Geometry check sheet. Reference: the model listing, model coordinates, mm. A direction names the side the tool comes from. Coordinates: 2 decimals unless noted, no trailing zeros. Write each loop counter-clockwise with the first axis right and the second up, starting at its lowest first coordinate (ties: lowest second). Pieces come first, ordered by that corner, then holes. Notation, with made-up numbers: M 43,-11 L 72,-11 A15 ccw 72,-2 Z; hole C -9.75,74 d11. An arc over 180 degrees is marked long. Write item = value, one per line. Start each with the question number.
```python
from build123d import *

# Parameters (mm, degrees)
BOSS_EXTRUDE1_DEPTH                        = 10
SKETCH3_R                                  = 4.5
CUT_EXTRUDE1_DEPTH                         = 44.28394626
MIRROR1_AT_THE_SECOND_PLANE_COPY_1_SKETC_R = 4.5
MIRROR1_AT_THE_SECOND_PLANE_COPY_1_DEPTH   = 44.28394626


with BuildPart() as part:
    # Sketch1 → Revolve1 (revolve)
    with BuildSketch(Plane.XY, mode=Mode.PRIVATE) as revolve1_sk:
        with BuildLine():
            Line((0, 9.5), (3.481747944, 9.5))
            ThreePointArc((3.481747944, 9.5), (3.98343056, 9.436056443), (4.453033806, 9.248314552))
            Line((4.453033806, 9.248314552), (7.6, 7.5))
            Line((7.6, 7.5), (7.6, -4.5))
            Line((7.6, -4.5), (17, -4.5))
            Line((17, -4.5), (17, -9.5))
            Line((17, -9.5), (7.6, -9.5))
            Line((7.6, -9.5), (0, -9.5))
            Line((0, -9.5), (0, 9.5))
        make_face()
    revolve(revolve1_sk.sketch.rotate(Axis((0, 9.5, 0), (0, -1, 0)), 90), axis=Axis((0, 9.5, 0), (0, -1, 0)))

    # Sketch2 → Boss-Extrude1 (add)
    with BuildSketch(Plane.XZ.offset(9.5)):
        with BuildLine():
            Line((17.5, 27.5), (-17.5, 27.5))
            ThreePointArc((-17.5, 27.5), (-24.571067812, 24.571067812), (-27.5, 17.5))
            Line((-27.5, 17.5), (-27.5, -17.5))
            ThreePointArc((-27.5, -17.5), (-24.571067812, -24.571067812), (-17.5, -27.5))
            Line((-17.5, -27.5), (17.5, -27.5))
            ThreePointArc((17.5, -27.5), (24.571067812, -24.571067812), (27.5, -17.5))
            Line((27.5, -17.5), (27.5, 17.5))
            ThreePointArc((27.5, 17.5), (24.571067812, 24.571067812), (17.5, 27.5))
        make_face()
    extrude(amount=BOSS_EXTRUDE1_DEPTH)

    # Sketch3 → Cut-Extrude1 (cut, through all)
    with BuildSketch(Plane(origin=(0, -9.5, 0), x_dir=(1, 0, 0), z_dir=(0, 1, 0))):
        with Locations(Location((-17.5, 17.5, 0), (0, 0, 270))):
            Circle(SKETCH3_R)
    cut_extrude1 = extrude(amount=-CUT_EXTRUDE1_DEPTH, mode=Mode.SUBTRACT)

    # Mirror1: Cut-Extrude1 across plane
    add(cut_extrude1.mirror(Plane.XY), mode=Mode.SUBTRACT)

    # Mirror1 at the second plane: Cut-Extrude1 across plane
    add(cut_extrude1.mirror(Plane(origin=(0, 0, 0), x_dir=(0, 0, 1), z_dir=(1, 0, 0))), mode=Mode.SUBTRACT)

    # Mirror1 at the second plane copy 1 sketc → Mirror1 at the second plane copy 1 (cut, through all)
    with BuildSketch(Plane(origin=(0, -9.5, 0), x_dir=(-1, 0, 0), z_dir=(0, 1, 0))):
        with Locations(Location((-17.5, 17.5, 0), (0, 0, 270))):
            Circle(MIRROR1_AT_THE_SECOND_PLANE_COPY_1_SKETC_R)
    extrude(amount=-MIRROR1_AT_THE_SECOND_PLANE_COPY_1_DEPTH, mode=Mode.SUBTRACT)


solid = part.part
```
Q1. Draft check along Z on faces 3 (the face through (-13.04, -14.43, 18.09)), 4 (the face through (-16.855, -7.035, -2.213)), 5 (the face through (-13, -9.5, -12)). Enter one of: pulls with the +Z half, pulls with the -Z half, needs draft (parallel to the pull), parting line crosses it, or undercut.
Q2. Scan lines: L1, parallel to Z at x = 17.5, y = -16.5; L2, parallel to Z at x = -15, y = -13.5. Record each from-to range of solid material in increasing order.
Q3. Cross-section at A-A on x = 19. Enter the section's corners in (y, z).
Q4. Gauge pin test, flat ends, axial feed: pin 1 (12 mm diameter, centred on x = 2.5, z = 11, fed in from +Y); pin 2 (12 mm diameter, centred on y = -2, z = -3.5, fed in from +X); pin 3 (1.5 mm diameter, centred on x = 5.5, y = -2.5, fed in from -Z); pin 4 (8 mm diameter, centred on x = -17.5, z = -17.5, fed in from +Y). Record the tip position at first contact, or that the pin passes through.
Q5. Cross-section at B-B on z = 0. Enter the section's corners in (x, y), and give its area (3 significant figures).
Q6. Cross-section at D-D on y = -7. Enter the section's corners in (x, z).
Q7. Cross-section at C-C on x = 0. Enter the section's corners in (y, z).
Q8. Set-up check for faces 1 (the face through (4, -4.5, -7)), 2 (the face through (24.65, -14.43, 24.49)): record each of +Z, -Z, +X, -X, +Y, -Y from which the full face is reachable in a straight line by a thin tool's end or side.
Values found:
q1.face_3 = undercut
q1.face_4 = parting line crosses it
q1.face_5 = needs draft
q2.L1 = -27.5 to -22, -13 to 13, 22 to 27.5
q2.L2 = -27.5 to -21.24, -13.76 to 13.76, 21.24 to 27.5
q3.outline = M -19.5,-27.39 L -9.5,-27.39 L -9.5,-21.74 L -19.5,-21.74 Z; M -19.5,-13.26 L -9.5,-13.26 L -9.5,13.26 L -19.5,13.26 Z; M -19.5,21.74 L -9.5,21.74 L -9.5,27.39 L -19.5,27.39 Z
q4.pin_1 = 8.79
q4.pin_2 = 17
q4.pin_3 = -5.93
q4.pin_4 = through
q5.outline = M -27.5,-19.5 L 27.5,-19.5 L 27.5,-9.5 L 17,-9.5 L 17,-4.5 L 7.6,-4.5 L 7.6,7.5 L 4.45,9.25 A2 ccw 3.48,9.5 L -3.48,9.5 A2 ccw -4.45,9.25 L -7.6,7.5 L -7.6,-4.5 L -17,-4.5 L -17,-9.5 L -27.5,-9.5 Z
q5.area = 926 mm²
q6.outline = C 0,0 d34
q7.outline = M -19.5,-27.5 L -9.5,-27.5 L -9.5,-17 L -4.5,-17 L -4.5,-7.6 L 7.5,-7.6 L 9.25,-4.45 A2 ccw 9.5,-3.48 L 9.5,3.48 A2 ccw 9.25,4.45 L 7.5,7.6 L -4.5,7.6 L -4.5,17 L -9.5,17 L -9.5,27.5 L -19.5,27.5 Z
q8.face_1 = +Y
q8.face_2 = +Z, +X, +Y, -Y
